Can you work these out from the drawing? Everything is in mm from the part's minimum corner. A direction names the side the tool comes from. Coordinates: 2 decimals unless noted, no trailing zeros. Loops run counter-clockwise (first coordinate to the right, second up) from the corner with the lowest first, then second, coordinate; pieces in that order, holes last.
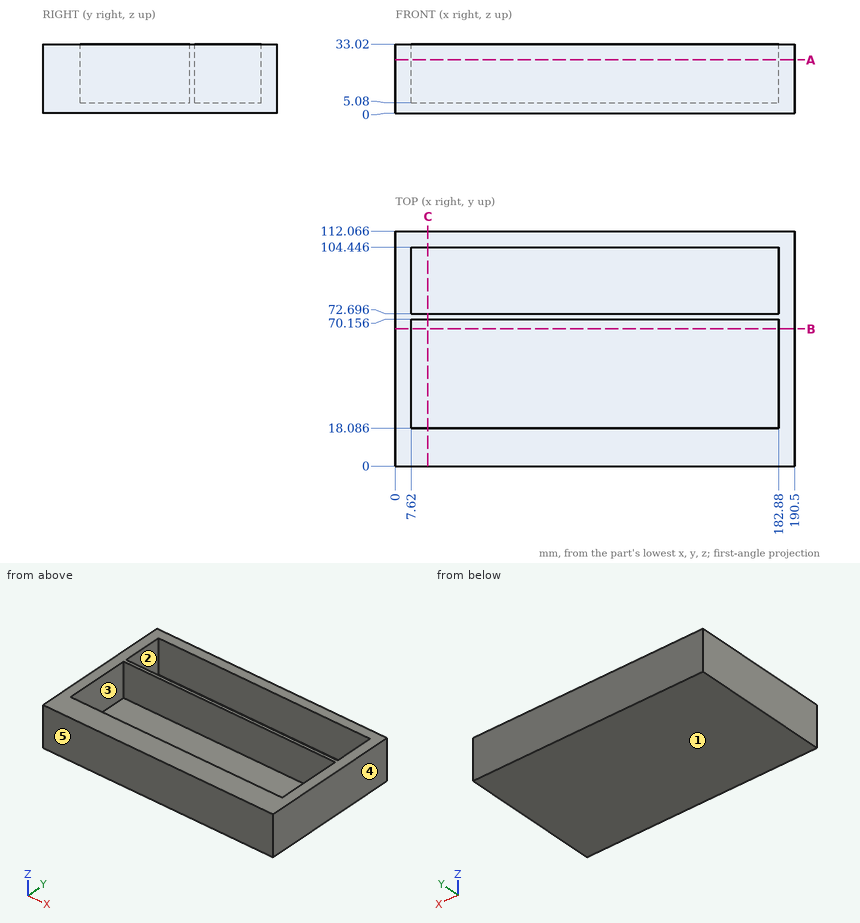
(1) Imagine slicing it at B-B, the plane y = 65.5. Write out the boundary of the cut face in (x, z), and give its area (3 significant figures).
Answers:
outline: (0, 0) - (190.5, 0) - (190.5, 33.02) - (182.88, 33.02) - (182.88, 5.08) - (7.62, 5.08) - (7.62, 33.02) - (0, 33.02) - close
area: 1,390 mm2
(2) For pin 1 (15.5 mm diameter, centred on x = 84, y = 32, fed in from +Z); pin 2 (8.5 mm diameter, centred on y = 39.5, z = 16.5, fed in from -X), each with a flat end and sliding along its axis, tell me the tip position at first contact or that it passes through.
Answers:
pin 1: stops at z = 5.08
pin 2: stops at x = 0
(3) We'd pull the mould along Y, two halves only. Please class the marked faces 3, 4 and 5: +Y half, -Y half, draft (parallel to the pull), parting line (faces both ways), or undercut.
Answers:
face 3: undercut
face 4: draft
face 5: -Y half
(4) Imagine slicing it at C-C, the plane x = 15.5. Write out the boundary of the cut face in (y, z).
Answers:
outline: (0, 0) - (112.07, 0) - (112.07, 33.02) - (104.45, 33.02) - (104.45, 5.08) - (72.7, 5.08) - (72.7, 33.02) - (70.16, 33.02) - (70.16, 5.08) - (18.09, 5.08) - (18.09, 33.02) - (0, 33.02) - close
(5) Which directions (+Z, -Z, +X, -X, +Y, -Y) give clear straight access to the entire face, cutting with the end or side of a thin tool? Please do the marked faces 1 and 2.
Answers:
face 1: -Z, +X, -X, +Y, -Y
face 2: +Z
(6) Imagine slicing it at A-A, the plane z = 25.5. Write out the boundary of the cut face in (x, y), and give its area (3 significant figures).
Answers:
outline: (0, 0) - (190.5, 0) - (190.5, 112.07) - (0, 112.07) - close; hole (7.62, 18.09) - (182.88, 18.09) - (182.88, 70.16) - (7.62, 70.16) - close; hole (7.62, 72.7) - (182.88, 72.7) - (182.88, 104.45) - (7.62, 104.45) - close
area: 6,660 mm2
(7) I need wall thicknesses on probe 1 along Y at (x, z) = (133.5, 21); probe 2 along X at (y, z) = (96.5, 28); probe 3 along Z at (x, y) = (15.5, 100). Which ranges of each line are inside material? Lowest first, please.
Answers:
probe 1: y = 0 to 18.09, 70.16 to 72.7, 104.45 to 112.07
probe 2: x = 0 to 7.62, 182.88 to 190.5
probe 3: z = 0 to 5.08
